Part model, mm, in its own coordinate system. Coordinates: 2 decimals unless noted, no trailing zeros. Write each loop counter-clockwise with the first axis right and the second up, starting at its lowest first coordinate (ties: lowest second). Pieces come first, ordered by that corner, then holes. Notation, with made-up numbers: (70.25, 49) -> (92.25, 49) arc R20 ccw to (92.25, 59) -> close; hole circle Ø6 at (-16, 54). An arc over 180 degrees is marked (long way). Write item = value, one per line. Start each with the question number.
Q1. Pin check, flat tip, straight feed: P1, Ø2, axis at x = 15, y = 0, coming from the +Z side. Stop position of the tip, or through.
Q2. Probe line 1 (Y direction, x = -15, z = 1.05); line 2 (X direction, y = -0.1, z = 0.5); line 3 (X direction, y = -1.05, z = 0.2). List the from-to ranges inside material, lowest first.
Q3. Band-saw the part on B-B, the plane y = 0. List the corners of the cut face in (x, z).
Q4. Band-saw the part on C-C, the plane z = 0.85. List the corners of the cut face in (x, y), plus the area to 3 significant figures.
Q5. Band-saw the part on A-A, the plane x = 30. List the corners of the cut face in (y, z).
from build123d import *

# Parameters (mm, degrees)
SKETCH_1_W          = 75
SKETCH_1_H          = 5
EXTRUDE_1_DEPTH     = 1.4
SKETCH_2_R          = 1.2
CUT_EXTRUDE_1_DEPTH = 51.4


with BuildPart() as part:
    # 草图1 → 凸台-拉伸1 (new body)
    with BuildSketch(Plane.XY):
        Rectangle(SKETCH_1_W, SKETCH_1_H)
    extrude(amount=EXTRUDE_1_DEPTH)

    # 草图2 → 切除-拉伸1 (cut)
    with BuildSketch(Plane.XY.offset(1.4)):
        with Locations((-30, 0)):
            Circle(SKETCH_2_R)
        with Locations((-15, 0)):
            Circle(SKETCH_2_R)
        Circle(SKETCH_2_R)
        with Locations((15, 0)):
            Circle(SKETCH_2_R)
        with Locations((30, 0)):
            Circle(SKETCH_2_R)
    extrude(amount=-CUT_EXTRUDE_1_DEPTH, mode=Mode.SUBTRACT)


solid = part.part
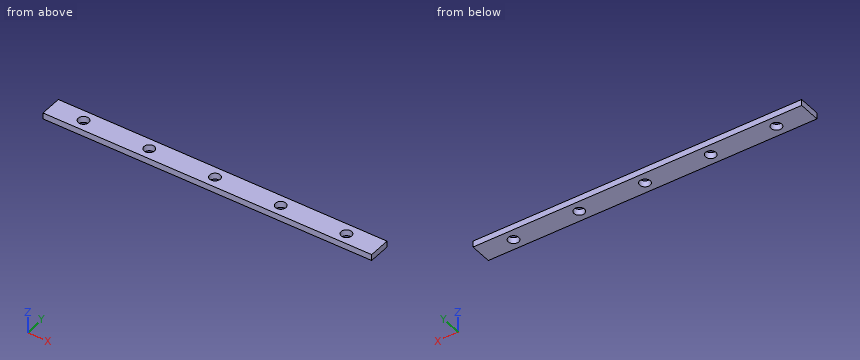
Ans:
q1.P1 = through
q2.line_1 = -2.5 to -1.2, 1.2 to 2.5
q2.line_2 = -37.5 to -31.2, -28.8 to -16.2, -13.8 to -1.2, 1.2 to 13.8, 16.2 to 28.8, 31.2 to 37.5
q2.line_3 = -37.5 to -30.58, -29.42 to -15.58, -14.42 to -0.58, 0.58 to 14.42, 15.58 to 29.42, 30.58 to 37.5
q3.outline = (-37.5, 0) -> (-31.2, 0) -> (-31.2, 1.4) -> (-37.5, 1.4) -> close; (-28.8, 0) -> (-16.2, 0) -> (-16.2, 1.4) -> (-28.8, 1.4) -> close; (-13.8, 0) -> (-1.2, 0) -> (-1.2, 1.4) -> (-13.8, 1.4) -> close; (1.2, 0) -> (13.8, 0) -> (13.8, 1.4) -> (1.2, 1.4) -> close; (16.2, 0) -> (28.8, 0) -> (28.8, 1.4) -> (16.2, 1.4) -> close; (31.2, 0) -> (37.5, 0) -> (37.5, 1.4) -> (31.2, 1.4) -> close
q4.outline = (-37.5, -2.5) -> (37.5, -2.5) -> (37.5, 2.5) -> (-37.5, 2.5) -> close; hole circle Ø2.4 at (-30, 0); hole circle Ø2.4 at (-15, 0); hole circle Ø2.4 at (0, 0); hole circle Ø2.4 at (15, 0); hole circle Ø2.4 at (30, 0)
q4.area = 352 mm2
q5.outline = (-2.5, 0) -> (-1.2, 0) -> (-1.2, 1.4) -> (-2.5, 1.4) -> close; (1.2, 0) -> (2.5, 0) -> (2.5, 1.4) -> (1.2, 1.4) -> close
